Source: CAD feature listing. Evaluate the final solid. Frame: model axes, mm. Face numbers are marked on the shaded views. A direction names the side the tool comes from. Give positions to 0.01 mm unless a question says otherwise; leave off trailing zeros. Write each loop counter-clockwise with the first axis right and the second up, starting at its lowest first coordinate (ties: lowest second). Pieces come first, ordered by that corner, then holes. Notation, with made-up numbers: M -35,89 L 0,89 A21 ccw 0,112 Z; hole C 76.25,48 d8. An arc over 180 degrees is marked long. Return JSON: item names as keys, results as strings.
```python
from build123d import *

# Parameters (mm, degrees)
SKETCH_1_R          = 18.68
SKETCH_1_R_2        = 15.652173913
EXTRUDE_2_DEPTH     = 2
SKETCH_1_4_R        = 23
SKETCH_1_4_R_2      = 1.25
SKETCH_1_4_R_3      = 18.68
EXTRUDE_3_DEPTH     = 8
EXTRUDE_4_DEPTH     = 8
SKETCH_3_R          = 1.8
CUT_EXTRUDE_1_DEPTH = 5
SKETCH_4_W          = 8
SKETCH_4_H          = 20
EXTRUDE_5_DEPTH     = 3


with BuildPart() as part:
    # Sketch 1 → Extrude 2 (new body)
    with BuildSketch(Plane(origin=(0, 0, 0), x_dir=(0, 0, -1), z_dir=(1, 0, 0))):
        Circle(SKETCH_1_R)
        Circle(SKETCH_1_R_2, mode=Mode.SUBTRACT)
    extrude(amount=EXTRUDE_2_DEPTH)

    # Sketch 1_4 → Extrude 3 (add)
    with BuildSketch(Plane(origin=(0, 0, 0), x_dir=(0, 0, -1), z_dir=(1, 0, 0))):
        Circle(SKETCH_1_4_R)
        with Locations((-7.940681222, 19.1705003)):
            Circle(SKETCH_1_4_R_2, mode=Mode.SUBTRACT)
        with Locations((-19.1705003, 7.940681222)):
            Circle(SKETCH_1_4_R_2, mode=Mode.SUBTRACT)
        with Locations((-19.1705003, -7.940681222)):
            Circle(SKETCH_1_4_R_2, mode=Mode.SUBTRACT)
        with Locations((-7.940681222, -19.1705003)):
            Circle(SKETCH_1_4_R_2, mode=Mode.SUBTRACT)
        with Locations((7.940681222, -19.1705003)):
            Circle(SKETCH_1_4_R_2, mode=Mode.SUBTRACT)
        with Locations((19.1705003, -7.940681222)):
            Circle(SKETCH_1_4_R_2, mode=Mode.SUBTRACT)
        with Locations((19.1705003, 7.940681222)):
            Circle(SKETCH_1_4_R_2, mode=Mode.SUBTRACT)
        with Locations((7.940681222, 19.1705003)):
            Circle(SKETCH_1_4_R_2, mode=Mode.SUBTRACT)
        Circle(SKETCH_1_4_R_3, mode=Mode.SUBTRACT)
    extrude(amount=EXTRUDE_3_DEPTH)

    # Sketch 2 → Extrude 4 (add)
    with BuildSketch(Plane.ZY):
        with BuildLine():
            Line((-23, -40.29), (-23, 0))
            ThreePointArc((-23, 0), (0, -23), (23, 0))
            Line((23, 0), (23, -40.29))
            Line((23, -40.29), (-23, -40.29))
        make_face()
    extrude(amount=-EXTRUDE_4_DEPTH)

    # Sketch 3 → Cut-Extrude 1 (cut)
    with BuildSketch(Plane.XZ.offset(40.29)):
        with Locations(Location((4, 19, 0), (0, 0, 270))):
            Circle(SKETCH_3_R)
    cut_extrude_1 = extrude(amount=-CUT_EXTRUDE_1_DEPTH, mode=Mode.SUBTRACT)

    # Mirror 1: Cut-Extrude 1 across plane
    add(cut_extrude_1.mirror(Plane(origin=(0, 0, 0), x_dir=(1, 0, 0), z_dir=(0, 0, -1))), mode=Mode.SUBTRACT)

    # Sketch 4 → Extrude 5 (add)
    with BuildSketch(Plane(origin=(0, -40.29, 0), x_dir=(-1, 0, 0), z_dir=(0, -1, 0))):
        with Locations((-4, 0)):
            Rectangle(SKETCH_4_W, SKETCH_4_H)
    extrude(amount=EXTRUDE_5_DEPTH)


solid = part.part
```
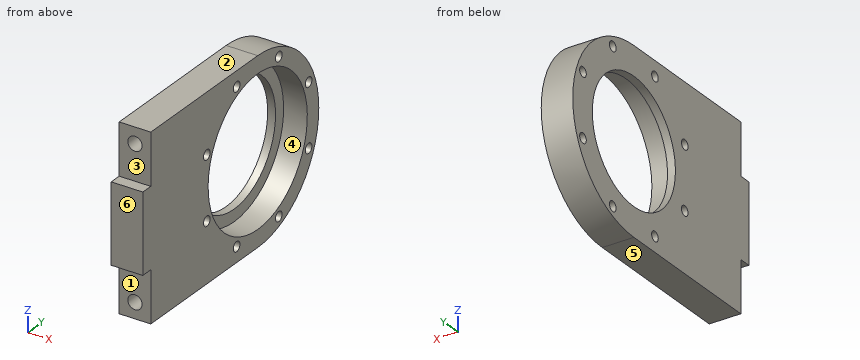
1) Draft query along Y for the marked faces 4, 5 and 6. Return one class per face: released by +Y, released by -Y, zero draft, split by the parting line, or undercut.
Numbers:
{"face 4": "undercut", "face 5": "zero draft", "face 6": "released by -Y"}
2) Set-up query: the marked faces 1, 2 and 3. Return all of +Z, -Z, +X, -X, +Y, -Y with unobstructed straight access to the full face (end or side cutting, diameter ignored); none if empty.
Numbers:
{"face 1": "-Z, +X, -X, -Y", "face 2": "+Z, +X, -X, +Y, -Y", "face 3": "+Z, +X, -X, -Y"}
3) Cut plane C-C, the plane x = 4. Give the number of separate pieces and of enclosed holes in the cut face, then the cut area to 3 significant figures.
Numbers:
{"separate pieces": "1", "enclosed holes": "9", "area": "1,570 mm²"}
4) Cut plane A-A, the plane z = 0. Return the cut outline in (x, y).
Numbers:
{"outline": "M 0,-43.29 L 8,-43.29 L 8,-18.68 L 2,-18.68 L 2,-15.65 L 0,-15.65 Z; M 0,15.65 L 2,15.65 L 2,18.68 L 8,18.68 L 8,23 L 0,23 Z"}
5) Cut plane D-D, the plane z = 16.5. Return the cut outline in (x, y).
Numbers:
{"outline": "M 0,-40.29 L 8,-40.29 L 8,-8.76 L 2,-8.76 L 2,8.76 L 8,8.76 L 8,16.02 L 0,16.02 Z"}
6) Cut plane B-B, the plane y = -3. Return the cut outline in (x, z), then the cut area to 3 significant figures.
Numbers:
{"outline": "M 0,-23 L 8,-23 L 8,-18.44 L 2,-18.44 L 2,-15.36 L 0,-15.36 Z; M 0,15.36 L 2,15.36 L 2,18.44 L 8,18.44 L 8,23 L 0,23 Z", "area": "85.3 mm²"}
7) Contact query for flat-ended pins moving along their axis: pin 1 Ø1.5 at (y, z) = (7.94, 19.17) entering from -X; pin 2 Ø1.8 at (x, z) = (4.5, 19.5) entering from -Y; pin 3 Ø3 at (x, z) = (4, -19) entering from +Y; pin 4 Ø3 at (x, z) = (4.5, -10) entering from +Y. Output: stop coordinate, or through.
Numbers:
{"pin 1": "passes through", "pin 2": "stops at y = -35.29", "pin 3": "stops at y = 14.92", "pin 4": "stops at y = 21.37"}
8) Line query: line 1 (Y direction, x = 4.75, z = -0.5); line 2 (Y direction, x = 4, z = -7.5); line 3 (Y direction, x = 1.75, z = -9). Output: solid intervals per line, ascending. Write a range as [from, to].
Numbers:
{"line 1": "y = [-43.29, -18.67], [18.67, 22.99]", "line 2": "y = [-43.29, -20.34], [-18, -17.11], [17.11, 18], [20.34, 21.74]", "line 3": "y = [-43.29, -19.83], [-18.51, -12.81], [12.81, 18.51], [19.83, 21.17]"}
